Drawing for the job (mm, zero at the part's lowest x, y, z). A direction names the side the tool comes from. Coordinates: 2 decimals unless noted, no trailing zeros. Write each loop counter-clockwise with the first axis right and the second up, starting at its lowest first coordinate (ties: lowest second). Pieces come first, ordered by that corner, then holes. Notation, with made-up numbers: M 30.5,2.25 L 65.5,2.25 A19 ccw 65.5,17.25 Z; hole C 89.5,-32.5 d9. An arc over 180 degrees is marked long. Use a Markdown table: item, result. Add a question column.
Q1. Slice it at B-B on z = 7.25. Write the cut outline in (x, y).
Q2. Slice it at D-D on z = 5. Write the cut outline in (x, y).
Q3. Pin check, flat tips, straight feed: pin 1 Ø1.1 at (x, y) = (0.5, 1) entering from +Z; pin 2 Ø0.8 at (x, y) = (0.5, 7.5) entering from +Z; pin 3 Ø0.5 at (x, y) = (0.5, 2) entering from -Z. Stop position of each tip, or through.
Q4. Wall check: L1, parallel to Y at x = 1.8, z = 2; L2, parallel to Y at x = 0.6, z = 3.5 (1 decimal); L3, parallel to Y at x = 0.9, z = 4 (1 decimal). Give the ranges that are in metal, low to high. Write a range as from..to.
Q5. Slice it at A-A on x = 0.2. Count the separate pieces of the cut face and the enclosed holes in it.
Q6. Tool access for the marked faces 1 and 2: list every direction of +Z, -Z, +X, -X, +Y, -Y with a clear straight run to the whole face (end or side of a thin tool).
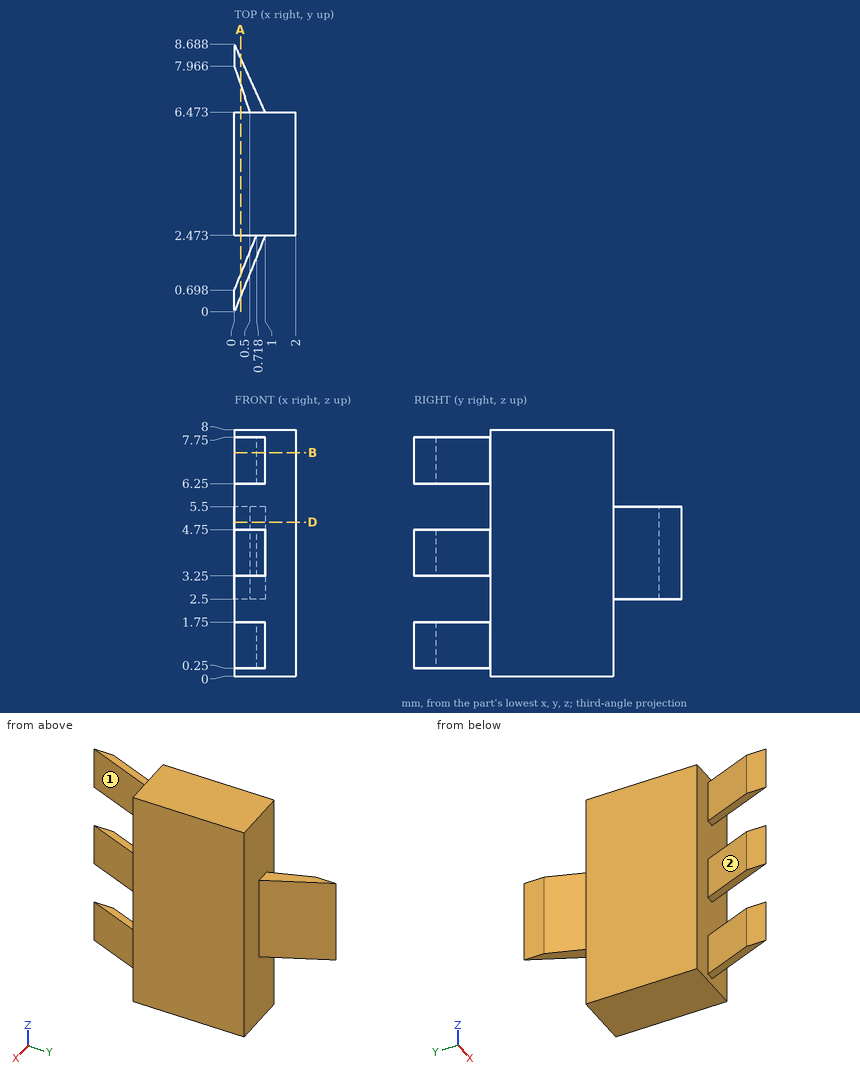
Recorded:
| question | item | result |
|---|---|---|
| 1 | outline | M 0,0 L 1,2.47 L 2,2.47 L 2,6.47 L 0,6.47 L 0,2.47 L 0.72,2.47 L 0,0.7 Z |
| 2 | outline | M 0,2.47 L 2,2.47 L 2,6.47 L 1,6.47 L 0,8.69 L 0,7.97 L 0.5,6.47 L 0,6.47 Z |
| 3 | pin 1 | z = 7.75 |
| 3 | pin 2 | z = 5.5 |
| 3 | pin 3 | z = 0.25 |
| 4 | L1 | 2.47..6.47 |
| 4 | L2 | 1.5..2.2, 2.5..7.4 |
| 4 | L3 | 2.2..6.7 |
| 5 | separate pieces | 5 |
| 5 | enclosed holes | 0 |
| 6 | face 1 | +Z, -Z, +X, -Y |
| 6 | face 2 | +Z, -Z, -X |
